```python
from build123d import *

# Parameters (mm, degrees)
F1_DEPTH = 50.8
F2_W     = 12.7
F2_H     = 12.7
F3_DEPTH = 12.7
F5_DEPTH = 25.4


with BuildPart() as f1:
    # F0 (on Top) → F1 (new body)
    with BuildSketch(Plane.XY):
        with BuildLine():
            Line((21.995319, 22.530525), (-3.404681, 22.530525))
            ThreePointArc((-3.404681, 22.530525), (-10.684751, 5.258633), (-28.804681, 0.464275))
            Line((-28.804681, 0.464275), (-28.804681, -21.601974))
            Line((-28.804681, -21.601974), (-1.992511, -21.601974))
            ThreePointArc((-1.992511, -21.601974), (2.643049, -2.569712), (21.995319, 0.464275))
            Line((21.995319, 0.464275), (21.995319, 22.530525))
        make_face()
    extrude(amount=F1_DEPTH)

    # F2 (on face) → F3 (cut)
    with BuildSketch(Plane(origin=(-28.804681, 0, 0), x_dir=(0, -1, 0), z_dir=(-1, 0, 0))):
        with Locations((15.251974, 44.45)):
            Rectangle(F2_W, F2_H)
    extrude(amount=-F3_DEPTH, mode=Mode.SUBTRACT)

    # F4 (on face) → F5 (cut)
    with BuildSketch(Plane(origin=(0, 22.530525, 0), x_dir=(-1, 0, 0), z_dir=(0, 1, 0))):
        with BuildLine():
            Line((-21.995319, 0), (-9.295319, 0))
            ThreePointArc((-9.295319, 0), (-6.407691, 17.318814), (-21.995319, 25.4))
            Line((-21.995319, 25.4), (-21.995319, 0))
        make_face()
    extrude(amount=-F5_DEPTH, mode=Mode.SUBTRACT)


solid = f1.part
```
Could you check a few things on this model? Use its own coordinates, in mm. A direction names the side the tool comes from. Round coordinates to 2 decimals unless told otherwise and drop trailing zeros. Loops run counter-clockwise (first coordinate to the right, second up) from the corner with the lowest first, then second, coordinate; pieces in that order, holes last. Notation, with made-up numbers: (38.5, 51) - (85.5, 51) arc R12 cw to (85.5, 60) - close; hole circle Ø8 at (-36.5, 65). An arc over 180 degrees is marked (long way). Answer as CSV lines item,"result".
1. Please list where these lines run through material, in increasing order: line 1 along Y through (x, z) = (-24.5, 26); line 2 along X through (y, z) = (-15, 21); line 3 along Y through (x, z) = (-16.5, 4). Write a range as [from, to].
Filled in:
line 1,"y = [-21.6, 0.05]"
line 2,"x = [-28.8, -3.05]"
line 3,"y = [-21.6, 1.66]"
2. I want a section at C-C on x = -22.5. List the corners of the cut face in (y, z) for me, then the cut area to 3 significant figures.
Filled in:
outline,"(-21.6, 0) - (0.16, 0) - (0.16, 50.8) - (-8.9, 50.8) - (-8.9, 38.1) - (-21.6, 38.1) - close"
area,"944 mm^2"
3. I want a section at A-A on x = 6.5. List the corners of the cut face in (y, z) for me.
Filled in:
outline,"(0.13, 0) - (22.53, 0) - (22.53, 3.79) - (0.13, 3.79) - close; (0.13, 17.5) - (22.53, 17.5) - (22.53, 50.8) - (0.13, 50.8) - close"
4. For pin 1 Ø2 at (x, y) = (1, 12) entering from -Z; pin 2 Ø8 at (x, z) = (-16.5, 16.5) entering from +Y; pin 3 Ø4 at (y, z) = (-16, 46) entering from -X; pin 4 Ø8 at (x, z) = (13, 25.5) entering from -Y, each with a flat end and sliding along its axis, tell me the tip position at first contact or that it passes through.
Filled in:
pin 1,"stops at z = 0"
pin 2,"stops at y = 3.85"
pin 3,"stops at x = -16.1"
pin 4,"stops at y = 1.18"
5. I want a section at D-D on y = -18.5. List the corners of the cut face in (x, z) for me, then the cut area to 3 significant figures.
Filled in:
outline,"(-28.8, 0) - (-2.81, 0) - (-2.81, 50.8) - (-16.1, 50.8) - (-16.1, 38.1) - (-28.8, 38.1) - close"
area,"1,160 mm^2"
6. We'd pull the mould along Z, two halves only. Please class faces 3 (the face through (-28.805, -10, 25)), 4 (the face through (-23, -15, 38.1)), 5 (the face through (6.3, 11, 17.1)), 6 (the face through (-10, -4, 0)): +Z half, -Z half, draft (parallel to the pull), parting line (faces both ways), or undercut.
Filled in:
face 3,"draft"
face 4,"+Z half"
face 5,"undercut"
face 6,"-Z half"
7. On a 3-axis mill with a long thin cutter (end or side, diameter ignored), from which of +Z, -Z, +X, -X, +Y, -Y can I reach the whole of each face in a straight line? I mean faces 1 (the face through (2, 1, 50.8)), 2 (the face through (-23, -8.902, 44)). Say none if no direction works.
Filled in:
face 1,"+Z, +X, -X, +Y, -Y"
face 2,"+Z, -X, -Y"
8. I want a section at B-B on z = 40.5. List the corners of the cut face in (x, y) for me, then the cut area to 3 significant figures.
Filled in:
outline,"(-28.8, -8.9) - (-16.1, -8.9) - (-16.1, -21.6) - (-1.99, -21.6) arc R17.65 cw to (22, 0.46) - (22, 22.53) - (-3.4, 22.53) arc R21.26 cw to (-28.8, 0.46) - close"
area,"1,090 mm^2"
